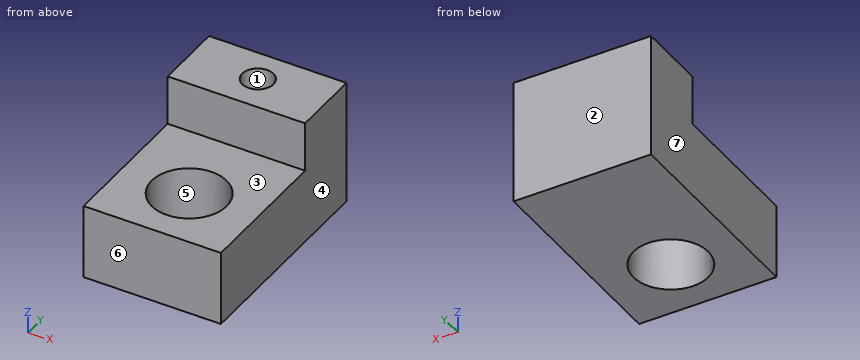
from build123d import *

# Parameters (mm, degrees)
SKETCH1_W                    = 5.5
SKETCH1_H                    = 8.5
BOSS_EXTRUDE1_DEPTH          = 3
SKETCH4_R                    = 1.5
CUT_EXTRUDE1_DEPTH           = 10
SKETCH7_W                    = 5.5
SKETCH7_H                    = 2.8
BOSS_EXTRUDE2_DEPTH          = 5
M1_6X0_35_TAPPED_HOLE1_D     = 1.25
M1_6X0_35_TAPPED_HOLE1_DEPTH = 4
M1_6X0_35_TAPPED_HOLE1_TIP   = 0.375537887


with BuildPart() as part:
    # Sketch1 → Boss-Extrude1 (new body)
    with BuildSketch(Plane.XY):
        Rectangle(SKETCH1_W, SKETCH1_H)
    extrude(amount=BOSS_EXTRUDE1_DEPTH)

    # Sketch4 → Cut-Extrude1 (cut)
    with BuildSketch(Plane.XY.offset(3)):
        with Locations((0, -1.75)):
            Circle(SKETCH4_R)
    extrude(amount=-CUT_EXTRUDE1_DEPTH, mode=Mode.SUBTRACT)

    # Sketch7 → Boss-Extrude2 (add)
    with BuildSketch(Plane(origin=(0, 0, 0), x_dir=(-1, 0, 0), z_dir=(0, 0, -1))):
        with Locations((0, 2.85)):
            Rectangle(SKETCH7_W, SKETCH7_H)
    extrude(amount=-BOSS_EXTRUDE2_DEPTH)

    # M1.6x0.35 Tapped Hole1
    with Locations(Plane.XY.offset(5)):
        with Locations((0, 2.9)):
            Hole(M1_6X0_35_TAPPED_HOLE1_D / 2, depth=M1_6X0_35_TAPPED_HOLE1_DEPTH)
            with Locations((0, 0, -(M1_6X0_35_TAPPED_HOLE1_DEPTH + M1_6X0_35_TAPPED_HOLE1_TIP / 2))):  # 118° drill point
                Cone(0, M1_6X0_35_TAPPED_HOLE1_D / 2, M1_6X0_35_TAPPED_HOLE1_TIP, mode=Mode.SUBTRACT)


solid = part.part
Design review of the part built by this model. Coordinates are the model's own, in mm. Face numbers are marked on the shaded views. A direction names the side the tool comes from. Give positions to 0.01 mm unless a question says otherwise; leave off trailing zeros. Loops run counter-clockwise (first coordinate to the right, second up) from the corner with the lowest first, then second, coordinate; pieces in that order, holes last. Notation, with made-up numbers: (-21, -31.75) -> (-6, -31.75) arc R16 cw to (-6, -14.75) -> close; hole circle Ø8 at (50, 1.25). An arc over 180 degrees is marked (long way). One line per question, with ' | ' between items. Start each with the question number.
(1) We need section B-B (z = 1.55). State the section outline as (x, y) points (3 decimals).
(2) For line 1 (Y direction, x = 0, z = 1.7) (3 decimals); line 2 (Y direction, x = -0.4, z = 1.2); line 3 (X direction, y = 2.9, z = 4.2) (3 decimals), list the stretches that pass through material, from the lowest coordinate up.
(3) Draft analysis for pull direction X (two halves, no side actions). For the marked faces 4, 5, 6 and 7, state which applies: +X half, -X half, draft (parallel to the pull), parting line (faces both ways), or undercut.
(4) We need section A-A (y = -1.75). State the section outline as (x, z) points, and give its area (3 significant figures).
(5) For the marked faces 1, 2 and 3, list the 3-axis set-ups (+Z, -Z, +X, -X, +Y, -Y) from which the entire face can be reached by the end or side of a thin tool; tool diameter is ignored.
(6) We need section D-D (z = 3.1). State the section outline as (x, y) points (3 decimals).
(7) Insertion check: P1, Ø3, axis at x = 0, y = -2, coming from the +Z side; P2, Ø1.8, axis at x = 0, y = -1.75, coming from the +Z side. Each pin has a flat end and moves straight along its axis. Give the tip position at first contact, or say it passes through.
(8) We need section C-C (x = 1.05). State the section outline as (y, z) points.
The answers:
1) outline: (-2.75, -4.25) -> (2.75, -4.25) -> (2.75, 4.25) -> (-2.75, 4.25) -> close; hole circle Ø3 at (0, -1.75); hole circle Ø1.25 at (0, 2.9)
2) line 1: y = -4.25 to -3.25, -0.25 to 2.275, 3.525 to 4.25 | line 2: y = -4.25 to -3.2, -0.3 to 2.42, 3.38 to 4.25 | line 3: x = -2.75 to -0.625, 0.625 to 2.75
3) face 4: +X half | face 5: undercut | face 6: draft | face 7: -X half
4) outline: (-2.75, 0) -> (-1.5, 0) -> (-1.5, 3) -> (-2.75, 3) -> close; (1.5, 0) -> (2.75, 0) -> (2.75, 3) -> (1.5, 3) -> close | area: 7.50 mm^2
5) face 1: +Z | face 2: +Z, -Z, +X, -X, +Y | face 3: +Z, +X, -X, -Y
6) outline: (-2.75, 1.45) -> (2.75, 1.45) -> (2.75, 4.25) -> (-2.75, 4.25) -> close; hole circle Ø1.25 at (0, 2.9)
7) P1: stops at z = 3 | P2: passes through
8) outline: (-4.25, 0) -> (-2.82, 0) -> (-2.82, 3) -> (-4.25, 3) -> close; (-0.68, 0) -> (4.25, 0) -> (4.25, 5) -> (1.45, 5) -> (1.45, 3) -> (-0.68, 3) -> close
